Geometry check sheet. Reference: the model listing, model coordinates, mm. Coordinates: 2 decimals unless noted, no trailing zeros. Order: outer loops, then holes, each group sorted by start corner. A loop starts at its lowest first (then second) coordinate and runs counter-clockwise, first axis right, second up. Notation, with made-up numbers: (82, 58.5) - (103, 58.5) arc R31 cw to (103, 88.5) - close; hole circle Ø5 at (-14, -35.75). An arc over 180 degrees is marked (long way). One line per item, written item: value. Start each with the question number.
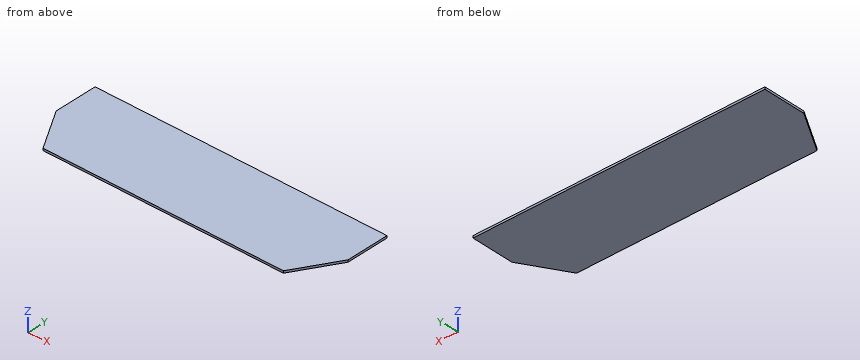
Autodesk Inventor part; units mm, degrees
ref_plane "YZ Plane" through (0, 0, 0) normal (1, 0, 0) x (0, 1, 0)
ref_plane "XZ Plane" through (0, 0, 0) normal (0, 1, 0) x (-1, 0, 0)
ref_plane "XY Plane" through (0, 0, 0) normal (0, 0, 1) x (1, 0, 0)
sketch "Sketch1" plane through (0, 0, 0) normal (0, 0, 1) x (1, 0, 0)
  line L0 (-206.5357, 101.3775) -> (225.2643, 101.3775)
  line L1 (225.2643, 101.3775) -> (225.2643, 37.8775)
  line L2 (225.2643, 37.8775) -> (187.1643, -25.6225)
  line L3 (187.1643, -25.6225) -> (-168.4357, -25.6225)
  line L4 (-168.4357, -25.6225) -> (-206.5357, 37.8775)
  line L5 (-206.5357, 37.8775) -> (-206.5357, 101.3775)
  point P0 (0, 0)
  dimension "d0" = 431.8
  dimension "d1" = 355.6
  dimension "d2" = 63.5
  dimension "d3" = 90
  dimension "d5" = 63.5
  dimension "d7" = 63.5
extrude "Extrusion1" add sketch "Sketch1" along normal blind 3.175
properties part number "Inner Plate"
Q1. Cross-section at C-C, the plane y = 16.5. Enter the section's corners in (x, z) (3 decimals), and give its area (3 significant figures).
Q2. Cross-section at B-B, the plane y = -5. Enter the section's corners in (x, z) (3 decimals), and give its area (3 significant figures).
Q3. Cross-section at A-A, the plane z = 1.7. Enter the section's corners in (x, y).
Q4. Gauge pin test, flat ends, axial feed: P1, Ø1, axis at y = -0.5, z = 2.5, coming from the +X side; P2, Ø1, axis at y = -9.5, z = 2.5, coming from the +X side. Record the tip position at first contact, or that the pin passes through.
Q5. Material ranges on probe 1 along X at (y, z) = (13.5, 1.7); probe 2 along X at (y, z) = (3.5, 1.3); probe 3 along Y at (x, z) = (189.5, 1.85), recorded low to high.
Check result:
1. outline: (-193.709, 0) - (212.438, 0) - (212.438, 3.175) - (-193.709, 3.175) - close
1. area: 1,290 mm2
2. outline: (-180.809, 0) - (199.538, 0) - (199.538, 3.175) - (-180.809, 3.175) - close
2. area: 1,210 mm2
3. outline: (-206.54, 37.88) - (-168.44, -25.62) - (187.16, -25.62) - (225.26, 37.88) - (225.26, 101.38) - (-206.54, 101.38) - close
4. P1: stops at x = 202.54
4. P2: stops at x = 197.14
5. probe 1: x = -191.91 to 210.64
5. probe 2: x = -185.91 to 204.64
5. probe 3: y = -21.73 to 101.38
